Read the model definition and answer for the solid it produces. Units are mm, in the model's axes. Face numbers are marked on the shaded views. A direction names the side the tool comes from. Coordinates: 2 decimals unless noted, no trailing zeros. Loops run counter-clockwise (first coordinate to the right, second up) from the corner with the lowest first, then second, coordinate; pieces in that order, holes last. Notation, with made-up numbers: (36, -6) -> (83, -6) arc R27 ccw to (83, 12) -> close; hole circle Ø7 at (40.25, -6.75). An arc over 180 degrees is marked (long way). Answer as a JSON object with one key per item and string values. Group by question number.
1) Section A-A, the plane z = 4.5 is taken. Give the vertices of the cut face in (x, y).
2) Section C-C, the plane y = 7 is taken. Give the vertices of the cut face in (x, z).
3) Determine the mould class of the marked faces 1, 2 and 3 for opening direction X: released by +X, released by -X, zero draft, split by the parting line, or undercut.
4) Flat-ended cylindrical pins translate along their axes: P1, Ø10, axis at x = -0.5, z = 127.5, coming from the -Y side; P2, Ø16, axis at x = 0, z = 120, coming from the -Y side; P3, Ø10, axis at y = 7.5, z = 20, coming from the +X side; P4, Ø4, axis at x = -15.5, z = 36, coming from the +Y side. Find the tip coordinate at first contact, or state that the pin passes through.
5) Consider probe 1 along X at (y, z) = (57, 120); probe 2 along Z at (x, y) = (0, 73.6); probe 3 along Y at (x, z) = (-20, 123). Determine where each line is inside the solid, lowest interval first. Write a range as [from, to].
6) Section B-B, the plane x = 2 is taken. Give the vertices of the cut face in (y, z).
7) Which of the six approach directions +Z, -Z, +X, -X, +Y, -Y give full straight-line access (tool end or side, diameter ignored) to the marked faces 4, 5 and 6?
8) Section D-D, the plane z = 78 is taken. Give the vertices of the cut face in (x, y), plus the area to 3 significant figures.
from build123d import *

# Parameters (mm, degrees)
F0_R     = 7.5
F0_W     = 60
F0_H     = 20
F1_DEPTH = 20
F2_DEPTH = 70
F3_W     = 28
F3_H     = 5
F3_W_2   = 6
F3_H_2   = 15
F3_W_3   = 1
F3_W_4   = 9
F3_H_3   = 10
F5_DEPTH = 30
F6_DEPTH = 5


with BuildPart() as f1:
    # F0 (on Front) → F1 (new body)
    with BuildSketch(Plane.XZ):
        with BuildLine():
            Line((-20, 30), (-20, 0))
            ThreePointArc((-20, 0), (0, -20), (20, 0))
            Line((20, 0), (20, 30))
            ThreePointArc((20, 30), (22.9289321881, 37.0710678119), (30, 40))
            Line((30, 40), (-30, 40))
            ThreePointArc((-30, 40), (-22.9289321881, 37.0710678119), (-20, 30))
        make_face()
        Circle(F0_R, mode=Mode.SUBTRACT)
        with Locations((0, 50)):
            Rectangle(F0_W, F0_H)
    extrude(amount=-F1_DEPTH)

    # F0 (on Front) → F2 (join)
    with BuildSketch(Plane.XZ):
        with Locations((0, 50)):
            Rectangle(F0_W, F0_H)
    extrude(amount=-F2_DEPTH)



with BuildPart() as f4:
    # F3 (on Right) → F4 (revolve)
    with BuildSketch(Plane.YZ):
        with Locations((55, 132.5)):
            Rectangle(F3_W, F3_H)
        with Locations((38, 142.5)):
            Rectangle(F3_W_2, F3_H_2)
        with Locations((72, 142.5)):
            Rectangle(F3_W_2, F3_H_2)
        with Locations((55, 142.5)):
            Rectangle(F3_W, F3_H_2)
    revolve(axis=Axis((0, 55, 120), (0, 1, 0)))


with BuildPart() as f1_1:
    add(f1.part)

    add(f4.part)  # F5 merges F4
    # F3 (on Right) → F5 (join, symmetric)
    with BuildSketch(Plane.YZ):
        Polygon((60, 90), (60, 60), (70, 60), (70, 90), (69, 90), align=None)
        with Locations((69.5, 97.5)):
            Rectangle(F3_W_3, F3_H_2)
        with Locations((64.5, 107.5)):
            Rectangle(F3_W_4, F3_H)
        with Locations((64.5, 115)):
            Rectangle(F3_W_4, F3_H_3)
        with Locations((64.5, 97.5)):
            Rectangle(F3_W_4, F3_H_2)
        with Locations((69.5, 115)):
            Rectangle(F3_W_3, F3_H_3)
        with Locations((69.5, 107.5)):
            Rectangle(F3_W_3, F3_H)
    extrude(amount=F5_DEPTH, both=True)

    # F3 (on Right) → F6 (join, symmetric)
    with BuildSketch(Plane.YZ):
        Polygon((35, 90), (0, 60), (60, 60), (60, 90), (41, 90), align=None)
        Polygon((41, 95.1428036188), (35, 90), (41, 90), align=None)
        Polygon((41, 90), (60, 90), (60, 105), (52.5001821322, 105), (41, 95.1428036188), align=None)
    extrude(amount=F6_DEPTH, both=True)

    # F3 (on Right) → F7 (revolve, cut)
    with BuildSketch(Plane.YZ):
        Polygon((35, 135), (35, 120), (41, 120), (41, 130), (41, 135), align=None)
        Polygon((41, 130), (41, 120), (60, 120), (69, 120), (69, 130), align=None)
        Polygon((69, 120), (70, 120), (75, 120), (75, 130), (69, 130), align=None)
        with Locations((72, 132.5)):
            Rectangle(F3_W_2, F3_H)
    revolve(axis=Axis((0, 55, 120), (0, 1, 0)), mode=Mode.SUBTRACT)


solid = f1_1.part
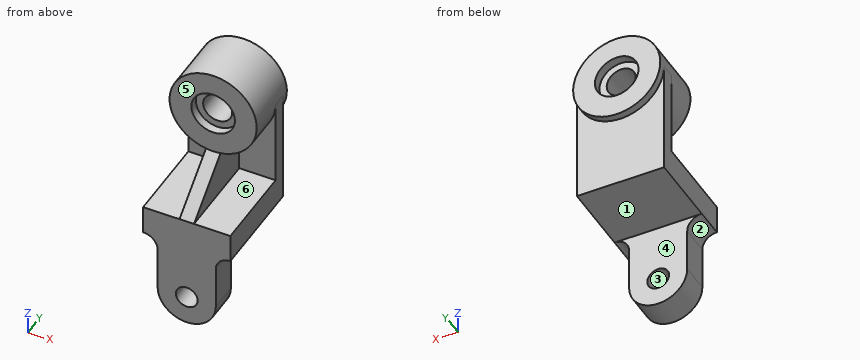
Determined:
{
 "1": {"outline": "(-20, 0) -> (-6, 0) -> (-6, 20) -> (-20, 20) -> close; (6, 0) -> (20, 0) -> (20, 20) -> (6, 20) -> close"},
 "2": {"outline": "(-30, 40) arc R10 cw to (-20, 30) -> (-20, 0) arc R20 ccw to (20, 0) -> (20, 30) arc R10 cw to (30, 40) -> (30, 60) -> (5, 60) -> (5, 66) -> (-5, 66) -> (-5, 60) -> (-30, 60) -> close; hole circle Ø15 at (0, 0)"},
 "3": {"face 1": "zero draft", "face 2": "released by -X", "face 3": "undercut"},
 "4": {"P1": "y = 41", "P2": "through", "P3": "x = 20", "P4": "y = 20"},
 "5": {"probe 1": "[-30, -10], [10, 30]", "probe 2": "[90, 105], [135, 150]", "probe 3": "[35, 75]"},
 "6": {"outline": "(0, -19.9) -> (20, -19.9) -> (20, -7.23) -> (0, -7.23) -> close; (0, 7.23) -> (20, 7.23) -> (20, 40) -> (70, 40) -> (70, 90.07) -> (75, 90.07) -> (75, 105.13) -> (69, 105.13) -> (69, 110.2) -> (41, 110.2) -> (41, 105.13) -> (35, 105.13) -> (35, 90.07) -> (35.08, 90.07) -> (35, 90) -> (0, 60) -> close; (35, 134.87) -> (41, 134.87) -> (41, 129.8) -> (69, 129.8) -> (69, 134.87) -> (75, 134.87) -> (75, 149.93) -> (35, 149.93) -> close"},
 "7": {"face 4": "-Z, +X, -X, +Y", "face 5": "+Z, +X, -X, -Y", "face 6": "+X, -Y"},
 "8": {"outline": "(-30, 60) -> (-5, 60) -> (-5, 21) -> (5, 21) -> (5, 60) -> (30, 60) -> (30, 70) -> (-30, 70) -> close", "area": "990 mm²"}
}
